```python
from build123d import *

# Parameters (mm, degrees)
F1_DEPTH = 63.5
F2_R     = 13.843
F3_DEPTH = 57.15
F4_R     = 3.175
F5_DEPTH = 6.35
F6_R     = 2.54
F7_DEPTH = 30.28857


with BuildPart() as f1:
    # F0 (on Front) → F1 (new body)
    with BuildSketch(Plane.XZ):
        with BuildLine():
            Line((15.143785, -4.7625), (15.143785, 4.7625))
            ThreePointArc((15.143785, 4.7625), (0, 15.875), (-15.143785, 4.7625))
            Line((-15.143785, 4.7625), (-15.143785, -4.7625))
            ThreePointArc((-15.143785, -4.7625), (0, -15.875), (15.143785, -4.7625))
        make_face()
    extrude(amount=F1_DEPTH)

    # F2 (on face) → F3 (cut)
    with BuildSketch(Plane.XZ.offset(63.5)):
        Circle(F2_R)
    extrude(amount=-F3_DEPTH, mode=Mode.SUBTRACT)

    # F4 (on face) → F5 (join)
    with BuildSketch(Plane(origin=(0, 0, 0), x_dir=(-1, 0, 0), z_dir=(0, 1, 0))):
        Circle(F4_R)
    extrude(amount=F5_DEPTH)

    # F6 (on face) → F7 (cut, through all)
    with BuildSketch(Plane(origin=(-15.143785, 0, 0), x_dir=(0, -1, 0), z_dir=(-1, 0, 0))):
        with Locations((12.7, 0)):
            Circle(F6_R)
        with Locations((50.8, 0)):
            Circle(F6_R)
        with Locations((25.4, 0)):
            Circle(F6_R)
        with Locations((38.1, 0)):
            Circle(F6_R)
    extrude(amount=-F7_DEPTH, mode=Mode.SUBTRACT)


solid = f1.part
```
Verification items for the finished model (mm, model axes). A direction names the side the tool comes from. Give positions to 0.01 mm unless a question says otherwise; leave off trailing zeros. Write each loop counter-clockwise with the first axis right and the second up, starting at its lowest first coordinate (ties: lowest second). Pieces come first, ordered by that corner, then holes. Notation, with made-up numbers: (46.25, 70) - (72.25, 70) arc R34 ccw to (72.25, 105) - close; hole circle Ø1 at (5, 23.25). An arc over 180 degrees is marked (long way). Put each result on its own line as item: value.
Q1. Mould release check, pull along Y, two halves, no side actions. Record for faces 1 (the face through (-15.144, -31, 0)), 2 (the face through (-14.387, -40.523, 0.763)), 3 (the face through (0, -6.35, 0)): released by +Y, released by -Y, zero draft, split by the parting line, or undercut.
Result:
face 1: zero draft
face 2: undercut
face 3: released by -Y
Q2. Section check C-C on z = 0. Count the separate pieces of the cut face and the enclosed holes in it, and give its area (3 significant figures).
Result:
separate pieces: 9
enclosed holes: 0
area: 328 mm2
Q3. Set-up check for faces 4 (the face through (-9, -63.5, 11)), 5 (the face through (7.4, -35.3, 11.7)), 6 (the face through (0.69, 3.13, -3.1)): record each of +Z, -Z, +X, -X, +Y, -Y from which the full face is reachable in a straight line by a thin tool's end or side.
Result:
face 4: +Z, -Z, +X, -X, -Y
face 5: -Y
face 6: +Y
Q4. Section check D-D on x = -8. Record the cut outline in (y, z).
Result:
outline: (-63.5, -13.71) - (0, -13.71) - (0, 13.71) - (-63.5, 13.71) - (-63.5, 11.3) - (-6.35, 11.3) - (-6.35, -11.3) - (-63.5, -11.3) - close
Q5. Scan lines: probe 1 along Y at (x, z) = (-14.7, 0); probe 2 along Z at (x, y) = (0, -8.5) (3 decimals); probe 3 along Y at (x, z) = (11, 4). Record each from-to range of solid material in increasing order. Write a range as from..to.
Result:
probe 1: -63.5..-53.34, -48.26..-40.64, -35.56..-27.94, -22.86..-15.24, -10.16..0
probe 2: -15.875..-13.843, 13.843..15.875
probe 3: -6.35..0
Q6. Depth check by flat-ended pin: P1, Ø1.5, axis at x = -5, z = -5, coming from the +Y side; P2, Ø8, axis at y = -45, z = 9, coming from the -X side; P3, Ø1.5, axis at x = 3, y = -31.5, coming from the +Z side; P4, Ø3, axis at y = -38.1, z = 0, coming from the -X side. Enter the tip coordinate at first touch or a pass-through.
Result:
P1: y = 0
P2: x = -15.07
P3: z = 15.71
P4: through
